```python
from build123d import *

# Parameters (mm, degrees)
SKETCH_1_W      = 59
SKETCH_1_H      = 58
SKETCH_1_R      = 3.3
EXTRUDE_1_DEPTH = 4
EXTRUDE_3_DEPTH = 3
EXTRUDE_START   = -3
EXTRUDE_6_DEPTH = 3
SKETCH_4_W      = 59
SKETCH_4_H      = 58
SKETCH_4_R      = 3.3
EXTRUDE_7_DEPTH = 4


with BuildPart() as part:
    # Эскиз1 → Бобышка-Вытянуть1 (new body)
    with BuildSketch(Plane.XY):
        Rectangle(SKETCH_1_W, SKETCH_1_H)
        with Locations((-15, 19)):
            Circle(SKETCH_1_R, mode=Mode.SUBTRACT)
        with Locations((15, 19)):
            Circle(SKETCH_1_R, mode=Mode.SUBTRACT)
        with BuildLine():
            Line((18.3, -14.2), (18.3, -1.3))
            ThreePointArc((18.3, -1.3), (15, 2), (11.7, -1.3))
            Line((11.7, -1.3), (11.7, -14.2))
            ThreePointArc((11.7, -14.2), (15, -17.5), (18.3, -14.2))
        make_face(mode=Mode.SUBTRACT)
        with BuildLine():
            Line((-18.3, -1.3), (-18.3, -14.2))
            ThreePointArc((-18.3, -14.2), (-15, -17.5), (-11.7, -14.2))
            Line((-11.7, -14.2), (-11.7, -1.3))
            ThreePointArc((-11.7, -1.3), (-15, 2), (-18.3, -1.3))
        make_face(mode=Mode.SUBTRACT)
    extrude(amount=EXTRUDE_1_DEPTH)

    # Эскиз5 → Бобышка-Вытянуть3 (add)
    with BuildSketch(Plane.ZY.offset(29.5)):
        with BuildLine():
            Line((0, 29), (7, 29))
            ThreePointArc((7, 29), (9.121320344, 28.121320344), (10, 26))
            Line((10, 26), (10, 25))
            Line((10, 25), (54, -19))
            Line((54, -19), (55, -19))
            ThreePointArc((55, -19), (57.121320344, -19.878679656), (58, -22))
            Line((58, -22), (58, -29))
            Line((58, -29), (0, -29))
            Line((0, -29), (0, 29))
        make_face()
    extrude(amount=-EXTRUDE_3_DEPTH)

    # Эскиз6 → Бобышка-Вытянуть6 (add)
    with BuildSketch(Plane(origin=(29.5, 0, 0), x_dir=(0, 0, -1), z_dir=(1, 0, 0)).offset(EXTRUDE_START)):
        with BuildLine():
            Line((0, 29), (0, -29))
            Line((0, -29), (-58, -29))
            Line((-58, -29), (-58, -22))
            ThreePointArc((-58, -22), (-57.121320344, -19.878679656), (-55, -19))
            Line((-55, -19), (-54, -19))
            Line((-54, -19), (-10, 25))
            Line((-10, 25), (-10, 26))
            ThreePointArc((-10, 26), (-9.121320344, 28.121320344), (-7, 29))
            Line((-7, 29), (0, 29))
        make_face()
    extrude(amount=EXTRUDE_6_DEPTH)

    # Эскиз4 → Бобышка-Вытянуть7 (add)
    with BuildSketch(Plane(origin=(0, -29, 0), x_dir=(-1, 0, 0), z_dir=(0, -1, 0))):
        with Locations((-5.17e-07, -29.000001301)):
            Rectangle(SKETCH_4_W, SKETCH_4_H)
        with Locations(Location((14.999999483, -48.000001301, 0), (0, 0, 270))):
            Circle(SKETCH_4_R, mode=Mode.SUBTRACT)
        with Locations(Location((-15.000000517, -48.000001301, 0), (0, 0, 270))):
            Circle(SKETCH_4_R, mode=Mode.SUBTRACT)
        with BuildLine():
            Line((11.699999483, -27.700001301), (11.699999483, -14.800001301))
            ThreePointArc((11.699999483, -14.800001301), (14.999999483, -11.500001301), (18.299999483, -14.800001301))
            Line((18.299999483, -14.800001301), (18.299999483, -27.700001301))
            ThreePointArc((18.299999483, -27.700001301), (14.999999483, -31.000001301), (11.699999483, -27.700001301))
        make_face(mode=Mode.SUBTRACT)
        with BuildLine():
            Line((-11.700000517, -14.800001301), (-11.700000517, -27.700001301))
            ThreePointArc((-11.700000517, -27.700001301), (-15.000000517, -31.000001301), (-18.300000517, -27.700001301))
            Line((-18.300000517, -27.700001301), (-18.300000517, -14.800001301))
            ThreePointArc((-18.300000517, -14.800001301), (-15.000000517, -11.500001301), (-11.700000517, -14.800001301))
        make_face(mode=Mode.SUBTRACT)
    extrude(amount=-EXTRUDE_7_DEPTH)


solid = part.part
```
Design review of the part built by this model. Coordinates are the model's own, in mm. A direction names the side the tool comes from. Round coordinates to 2 decimals unless told otherwise and drop trailing zeros. Write each loop counter-clockwise with the first axis right and the second up, starting at its lowest first coordinate (ties: lowest second). Pieces come first, ordered by that corner, then holes.
Item 1: For faces 1 (the flat face through (-6, -25, 35)), 2 (the flat face through (-18.3, -27, 21)), 3 (the cylindrical face through (-15.1, -17.5, 2)), 4 (the flat face through (0, 0, 0)), list the 3-axis set-ups (+Z, -Z, +X, -X, +Y, -Y) from which the entire face can be reached by the end or side of a thin tool; tool diameter is ignored.
Item 2: We need section B-B on x = 15. Write out the cut boundary in (y, z), and give its area (3 significant figures).
Item 3: We need section A-A on y = 19. Write out the cut boundary in (x, z).
Item 4: The part is to be moulded in two halves that separate along Z. For faces 5 (the cylindrical face through (14.01, -27.03, 51.15)), 6 (the flat face through (0, -29, 29)), 7 (the flat face through (-28, -23, 58)), say which applies: +Z half, -Z half, draft (parallel to the pull), parting line (faces both ways), or undercut.
Item 5: We need section C-C on z = 48. Write out the cut boundary in (x, y), and give its area (3 significant figures).
Item 6: For probe 1 along Y at (x, z) = (-15, 1.7); probe 2 along X at (y, z) = (-17.5, 42); probe 3 along Z at (x, y) = (-8.5, -17), list the stretches that pass through material, from the lowest coordinate up.
Item 7: Clearance check with flat-ended pins moving along their axes: pin 1 Ø2 at (x, z) = (18, 47.5) entering from +Y; pin 2 Ø0.5 at (x, y) = (27.5, 25.5) entering from +Z; pin 3 Ø4 at (x, y) = (-15, 19) entering from -Z; pin 4 Ø1.1 at (x, z) = (-28, 54.5) entering from +Y. State where each tip first meets the part, or that it passes through.
Item 8: We need section D-D on y = 5.5. Write out the cut boundary in (x, z).
Returned:
1. face 1: +Z, +Y
1. face 2: +Y, -Y
1. face 3: +Z, -Z
1. face 4: -Z, +X, -X, +Y, -Y
2. outline: (-29, 0) - (-17.5, 0) - (-17.5, 4) - (-25, 4) - (-25, 11.5) - (-29, 11.5) - close; (-29, 31) - (-25, 31) - (-25, 44.7) - (-29, 44.7) - close; (-29, 51.3) - (-25, 51.3) - (-25, 58) - (-29, 58) - close; (2, 0) - (15.7, 0) - (15.7, 4) - (2, 4) - close; (22.3, 0) - (29, 0) - (29, 4) - (22.3, 4) - close
2. area: 239 mm2
3. outline: (-29.5, 0) - (-18.3, 0) - (-18.3, 4) - (-26.5, 4) - (-26.5, 16) - (-29.5, 16) - close; (-11.7, 0) - (11.7, 0) - (11.7, 4) - (-11.7, 4) - close; (18.3, 0) - (29.5, 0) - (29.5, 16) - (26.5, 16) - (26.5, 4) - (18.3, 4) - close
4. face 5: undercut
4. face 6: draft
4. face 7: +Z half
5. outline: (-29.5, -29) - (-18.3, -29) - (-18.3, -25) - (-26.5, -25) - (-26.5, -13) - (-29.5, -13) - close; (-11.7, -29) - (11.7, -29) - (11.7, -25) - (-11.7, -25) - close; (18.3, -29) - (29.5, -29) - (29.5, -13) - (26.5, -13) - (26.5, -25) - (18.3, -25) - close
5. area: 255 mm2
6. probe 1: y = -29 to -17.5, 2 to 15.7, 22.3 to 29
6. probe 2: x = -29.5 to -26.5, 26.5 to 29.5
6. probe 3: z = 0 to 4
7. pin 1: stops at y = -25
7. pin 2: stops at z = 10
7. pin 3: passes through
7. pin 4: stops at y = -18.95
8. outline: (-29.5, 0) - (29.5, 0) - (29.5, 29.5) - (26.5, 29.5) - (26.5, 4) - (-26.5, 4) - (-26.5, 29.5) - (-29.5, 29.5) - close
